Autodesk Fusion 360 part; units mm, degrees
sketch "Boceto1" plane through (0, 0, 0) normal (0, 0, 1) x (1, 0, 0)
  line L0 (0, 35) -> (-2.3299, 29.9094)
  line L1 (0, 35) -> (2.3299, 29.9094)
  line L2 (-24.7487, 24.7487) -> (-19.5017, 22.7966)
  line L3 (-24.7487, 24.7487) -> (-22.7966, 19.5017)
  line L4 (-35, 0) -> (-29.9094, 2.3299)
  line L5 (-35, 0) -> (-29.9094, -2.3299)
  line L6 (-24.7487, -24.7487) -> (-22.7966, -19.5017)
  line L7 (-24.7487, -24.7487) -> (-19.5017, -22.7966)
  line L8 (0, -35) -> (-2.3299, -29.9094)
  line L9 (0, -35) -> (2.3299, -29.9094)
  line L10 (24.7487, -24.7487) -> (19.5017, -22.7966)
  line L11 (24.7487, -24.7487) -> (22.7966, -19.5017)
  line L12 (35, 0) -> (29.9094, -2.3299)
  line L13 (35, 0) -> (29.9094, 2.3299)
  line L14 (24.7487, 24.7487) -> (22.7966, 19.5017)
  line L15 (24.7487, 24.7487) -> (19.5017, 22.7966)
  arc A0 (-2.3299, 29.9094) -> (-19.5017, 22.7966) centre (0, 0) ccw
  arc A1 (19.5017, 22.7966) -> (2.3299, 29.9094) centre (0, 0) ccw
  arc A2 (29.9094, 2.3299) -> (22.7966, 19.5017) centre (0, 0) ccw
  arc A3 (22.7966, -19.5017) -> (29.9094, -2.3299) centre (0, 0) ccw
  arc A4 (2.3299, -29.9094) -> (19.5017, -22.7966) centre (0, 0) ccw
  arc A5 (-19.5017, -22.7966) -> (-2.3299, -29.9094) centre (0, 0) ccw
  arc A6 (-22.7966, 19.5017) -> (-29.9094, 2.3299) centre (0, 0) ccw
  arc A7 (-29.9094, -2.3299) -> (-22.7966, -19.5017) centre (0, 0) ccw
  dimension "d1" = 60
  dimension "d3" = 360
extrude "Extruir1" add sketch "Boceto1" against normal blind 85
Work out the finished part from the listing and answer in its coordinate system (mm). A direction names the side the tool comes from. Coordinates: 2 decimals unless noted, no trailing zeros. Loops run counter-clockwise (first coordinate to the right, second up) from the corner with the lowest first, then second, coordinate; pieces in that order, holes last.
1) Section A-A (z = -57) is taken. Give the vertices of the cut face in (x, y), plus the area to 3 significant figures.
Results:
outline: (-35, 0) - (-29.91, -2.33) arc R30 ccw to (-22.8, -19.5) - (-24.75, -24.75) - (-19.5, -22.8) arc R30 ccw to (-2.33, -29.91) - (0, -35) - (2.33, -29.91) arc R30 ccw to (19.5, -22.8) - (24.75, -24.75) - (22.8, -19.5) arc R30 ccw to (29.91, -2.33) - (35, 0) - (29.91, 2.33) arc R30 ccw to (22.8, 19.5) - (24.75, 24.75) - (19.5, 22.8) arc R30 ccw to (2.33, 29.91) - (0, 35) - (-2.33, 29.91) arc R30 ccw to (-19.5, 22.8) - (-24.75, 24.75) - (-22.8, 19.5) arc R30 ccw to (-29.91, 2.33) - close
area: 2,920 mm2
2) For faces 1 (the flat face through (22.2, 23.8, -41.9)), 2 (the flat face through (22.2, -23.8, -41.9)), 3 (the flat face through (23.8, 22.2, -41.9)), 4 (the cylindrical face through (-27.665, 11.603, -41.905)), determine the directions among +Z, -Z, +X, -X, +Y, -Y from which every point of the face is accessible in a straight line to the end or side of a thin tool.
Results:
face 1: +Z, -Z, +Y
face 2: +Z, -Z, -Y
face 3: +Z, -Z, +X
face 4: +Z, -Z, -X
3) Section B-B (x = -16) is taken. Give the vertices of the cut face in (y, z).
Results:
outline: (-25.38, -85) - (25.38, -85) - (25.38, 0) - (-25.38, 0) - close
4) Section C-C (y = -14.5) is taken. Give the vertices of the cut face in (x, z).
Results:
outline: (-26.26, -85) - (26.26, -85) - (26.26, 0) - (-26.26, 0) - close
5) Consider probe 1 along Y at (x, z) = (2.5, -55.5); probe 2 along Y at (x, z) = (4, -43.5). Determine where each line is inside the solid, lowest interval first.
Results:
probe 1: y = -29.9 to 29.9
probe 2: y = -29.73 to 29.73
6) Flat-ended cylindrical pins translate along their axes: pin 1 (3 mm diameter, centred on y = 4.5, z = -47.5, fed in from +X); pin 2 (4 mm diameter, centred on x = 8, z = -10, fed in from -Y); pin 3 (3 mm diameter, centred on y = -6.5, z = -43.5, fed in from +X). Find the tip coordinate at first contact, or state that the pin passes through.
Results:
pin 1: stops at x = 29.85
pin 2: stops at y = -29.39
pin 3: stops at x = 29.58
7) For a pull along Y with two mould halves and no side action, classify faces 5 (the flat face through (0, 0, 0)), 6 (the flat face through (-32.49, -1.15, -41.9)), 7 (the cylindrical face through (27.665, -11.603, -41.905)), 8 (the flat face through (-1.15, 32.49, -41.9)) as +Y half, -Y half, draft (parallel to the pull), parting line (faces both ways), or undercut.
Results:
face 5: draft
face 6: -Y half
face 7: undercut
face 8: +Y half
